Work out the finished part from the listing and answer in its coordinate system (mm). Face numbers are marked on the shaded views. Coordinates: 2 decimals unless noted, no trailing zeros. Order: outer loops, then holes, each group sorted by start corner. A loop starts at its lowest first (then second) coordinate and runs counter-clockwise, first axis right, second up. Notation, with made-up numbers: M -32.75,68.5 L 19.25,68.5 A19 ccw 19.25,72.5 Z; hole C 26,31.25 d5. An arc over 180 degrees is marked long. Answer in a Markdown table with one row per item. Add a question column.
Item 1: The part is cut by section A-A (x = -64). Write down the section's boundary in (y, z).
Item 2: The part is cut by section C-C (y = 7.25). Write down the section's boundary in (x, z).
Item 3: Consider line 1 (X direction, y = 8, z = 17.75); line 2 (X direction, y = 8, z = -22.5); line 3 (Y direction, x = -64, z = 19). Determine where each line is inside the solid, lowest interval first. Write a range as from..to.
Item 4: Flat-ended cylindrical pins translate along their axes: pin 1 Ø12 at (x, z) = (-50, -6) entering from -Y; pin 2 Ø5 at (y, z) = (13.5, 4.5) entering from -X; pin 3 Ø4 at (y, z) = (12.5, -7.5) entering from -X. Find the tip coordinate at first contact, or state that the pin passes through.
Item 5: The part is cut by section D-D (z = -10). Write down the section's boundary in (x, y).
Item 6: The mould has two halves that part along X. Classify the marked faces 1, 2, 3 and 4: released by +X, released by -X, zero draft, split by the parting line, or undercut.
Item 7: The part is cut by section B-B (z = 0). Write down the section's boundary in (x, y).
Autodesk Inventor part; units mm, degrees
ref_plane "YZ Plane" through (0, 0, 0) normal (1, 0, 0) x (0, 1, 0)
ref_plane "XZ Plane" through (0, 0, 0) normal (0, 1, 0) x (-1, 0, 0)
ref_plane "XY Plane" through (0, 0, 0) normal (0, 0, 1) x (1, 0, 0)
sketch "Skizze1" plane through (0, 0, 0) normal (0, 1, 0) x (-1, 0, 0)
  line L0 (10.0667, 24) -> (117.9333, 24)
  line L1 (117.9333, -24) -> (10.0667, -24)
  line L2 (0, 0) -> (128, 0) construction
  arc A0 (6.7408, 22.2222) -> (6.7408, -22.2222) centre (40, 0) ccw
  arc A1 (121.2592, -22.2222) -> (121.2592, 22.2222) centre (88, 0) ccw
  arc A2 (121.2592, 22.2222) -> (117.9333, 24) centre (117.9333, 20) ccw
  arc A3 (117.9333, -24) -> (121.2592, -22.2222) centre (117.9333, -20) ccw
  arc A4 (6.7408, -22.2222) -> (10.0667, -24) centre (10.0667, -20) ccw
  arc A5 (10.0667, 24) -> (6.7408, 22.2222) centre (10.0667, 20) ccw
  point P0 (120, -24)
  point P1 (120, -24)
  point P2 (120, -24)
  point P3 (120, 24)
  point P4 (120, 24)
  point P5 (120, 24)
  point P6 (8, -24)
  point P7 (8, -24)
  point P8 (8, -24)
  point P9 (8, 24)
  point P10 (8, 24)
  point P11 (8, 24)
  point P12 (128, 0)
  dimension "d1" = 0
  dimension "d3" = 0
  dimension "d2" = 48
  dimension "d24" = 128
  dimension "d25" = 4
  dimension "d26" = 40
  dimension "d27" = 40
extrude "Extrusion1" add sketch "Skizze1" along normal blind 16
sketch "Skizze2" plane through (0, 0, 0) normal (0, 1, 0) x (1, 0, 0)
  line L0 (-117.9333, -24) -> (-10.0667, -24)
  arc A0 (-121.2592, 22.2222) -> (-121.2592, -22.2222) centre (-88, 0) ccw
  point P0 (0, 0)
  point P1 (-64, 0)
  point P2 (2, 0)
  point P3 (-112, 0)
  point P4 (2, 0)
  point P5 (-128, 0)
  point P6 (-64, -24)
  dimension "d29" = 48
hole "Bohrung1" at (-64, 0, 0) direction (0, 1, 0) diameter 36 depth 16
hole "Bohrung2" at (-112, 0, 0) direction (0, 1, 0) diameter 16 depth 16
sketch "Skizze3" plane through (-10.0667, 0, -24) normal (0, 0, -1) x (-1, 0, 0)
  line L0 (0, 0) -> (0, 16)
  line L1 (111.1924, 0) -> (111.1924, 16)
  line L2 (0, 0) -> (107.8665, 0)
  point P0 (-10.0667, 0)
  point P1 (103.1924, 8)
  point P2 (0, 8)
  point P3 (53.9333, 8)
  point P4 (53.9333, 0)
  dimension "d37" = 8
hole "Bohrung3" at (-113.2592, 8, -24) direction (0, 0, 1) diameter 8 end through all
hole "Bohrung4" at (-64, 8, -24) direction (0, 0, 1) diameter 8 end through all
properties part number "wheel_support"
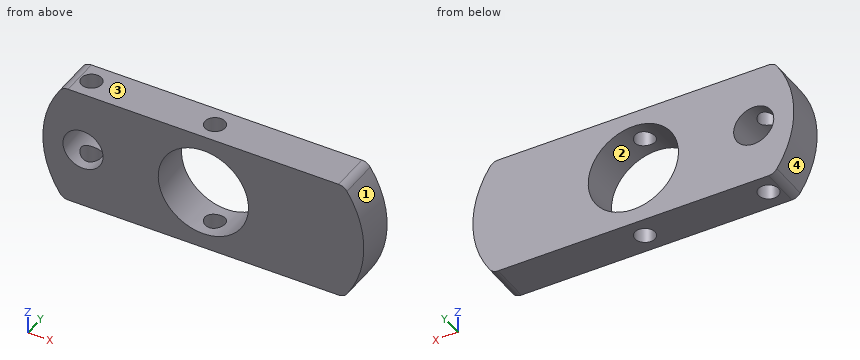
Reply:
| question | item | result |
|---|---|---|
| 1 | outline | M 0,-24 L 4,-24 L 4,-18 L 0,-18 Z; M 0,18 L 4,18 L 4,24 L 0,24 Z; M 12,-24 L 16,-24 L 16,-18 L 12,-18 Z; M 12,18 L 16,18 L 16,24 L 12,24 Z |
| 2 | outline | M -121.26,-22.22 A4 ccw -117.93,-24 L -117.19,-24 L -117.19,-6.09 A8 cw -117.19,6.09 L -117.19,24 L -117.93,24 A4 ccw -121.26,22.22 A40 ccw Z; M -109.33,-24 L -67.93,-24 L -67.93,-17.57 A18 cw -67.93,17.57 L -67.93,24 L -109.33,24 L -109.33,7.54 A8 cw -109.33,-7.54 Z; M -60.07,-24 L -10.07,-24 A4 ccw -6.74,-22.22 A40 ccw -6.74,22.22 A4 ccw -10.07,24 L -60.07,24 L -60.07,17.57 A18 cw -60.07,-17.57 Z |
| 3 | line 1 | x = -123.85..-117.26, -109.26..-68, -60..-4.15 |
| 3 | line 2 | x = -121.06..-117.26, -109.26..-68, -60..-6.94 |
| 3 | line 3 | y = 0..4, 12..16 |
| 4 | pin 1 | stops at y = 0 |
| 4 | pin 2 | stops at x = -127.95 |
| 4 | pin 3 | stops at x = -127.62 |
| 5 | outline | M -126.73,0 L -78.97,0 L -78.97,16 L -126.73,16 Z; M -49.03,0 L -1.27,0 L -1.27,16 L -49.03,16 Z; hole C -113.26,8 d8 |
| 6 | face 1 | released by +X |
| 6 | face 2 | undercut |
| 6 | face 3 | zero draft |
| 6 | face 4 | released by -X |
| 7 | outline | M -128,0 L -120,0 L -120,16 L -128,16 Z; M -104,0 L -82,0 L -82,16 L -104,16 Z; M -46,0 L 0,0 L 0,16 L -46,16 Z |
